Part model, mm, in its own coordinate system. A direction names the side the tool comes from. Coordinates: 2 decimals unless noted, no trailing zeros. Write each loop counter-clockwise with the first axis right and the second up, starting at its lowest first coordinate (ties: lowest second). Pieces come first, ordered by that corner, then holes. Notation, with made-up numbers: (36, -33) - (77, -33) arc R24 ccw to (77, -15) - close; hole circle Ø1 at (44.5, 5). An arc over 180 degrees is marked (long way). Use one line per item in the form item = value. Start each with the question number.
from build123d import *

# Parameters (mm, degrees)
BOSS_EXTRUDE1_START             = -487.984875
SKETCH3_R                       = 24.13
BOSS_EXTRUDE1_DEPTH             = 975.96975
CHAMFER1_SIZE                   = 0.254
BOSS_EXTRUDE3_REACH             = 985.674
SKETCH6_R                       = 24.13
SKETCH6_R_2                     = 22.352
BOSS_EXTRUDE3_DIRECTION_2_REACH = 985.674
BOSS_EXTRUDE2_DEPTH             = 508
BOSS_EXTRUDE2_DEPTH_BACK        = 508
LPATTERN1_COUNT                 = 2
LPATTERN1_PITCH                 = 33.02


with BuildPart() as part:
    # Sketch2 → Revolve1 (revolve)
    with BuildSketch(Plane.XY, mode=Mode.PRIVATE) as revolve1_sk:
        Polygon((-493.7125, 0), (-493.7125, 11.1125), (-495.096875, 11.1125), (-495.096875, 15.712927565), (-489.762875, 15.712927565), (-489.762875, 20.574), (-495.096875, 20.574), (-495.096875, 24.13), (-493.318875, 24.13), (-493.318875, 22.352), (-487.984875, 22.352), (-487.984875, 0), align=None)
    revolve(revolve1_sk.sketch.rotate(Axis((-493.7125, 0, 0), (1, 0, 0)), 180), axis=Axis((-493.7125, 0, 0), (1, 0, 0)))


with BuildPart() as body_2:
    # Mirror2: mirrored copy
    add(part.part.mirror(Plane(origin=(0, 0, 0), x_dir=(0, 0, 1), z_dir=(1, 0, 0))))


with BuildPart() as part_1:
    add(part.part)

    add(body_2.part)  # Boss-Extrude1 merges body 2
    # Sketch3 → Boss-Extrude1 (add)
    with BuildSketch(Plane(origin=(0, 0, 0), x_dir=(0, 0, -1), z_dir=(1, 0, 0)).offset(BOSS_EXTRUDE1_START)):
        with Locations(Location((0, 0, 0), (0, 0, 270))):
            Circle(SKETCH3_R)
    extrude(amount=BOSS_EXTRUDE1_DEPTH)

    # Chamfer1
    chamfer1_edges = [part_1.edges().sort_by_distance(p)[0] for p in [
        (493.318875, 24.13, 0),
        (-493.318875, 24.13, 0),
    ]]
    chamfer(chamfer1_edges, length=CHAMFER1_SIZE)

    # Boss-Extrude3: up to this face of the body (flat: up to its plane)
    boss_extrude3_end = Plane(part_1.part.faces().sort_by_distance((-493.318875, 23.20068474, 0))[0])
    # Sketch6 → Boss-Extrude3 (add, up to the picked face)
    with BuildSketch(Plane.ZY.offset(487.984875), mode=Mode.PRIVATE) as boss_extrude3_sk1:
        with Locations(Location((0, 0, 0), (0, 0, 270))):
            Circle(SKETCH6_R)
        Circle(SKETCH6_R_2, mode=Mode.SUBTRACT)
    boss_extrude3_tool1 = split(extrude(boss_extrude3_sk1.sketch, amount=BOSS_EXTRUDE3_REACH, mode=Mode.PRIVATE), bisect_by=boss_extrude3_end, keep=Keep.BOTH, mode=Mode.PRIVATE)
    add(boss_extrude3_tool1.solids().sort_by(Axis((-487.984875, 23.447501, 0), (-1, 0, 0)))[0])

    # Boss-Extrude3 direction 2: up to this face of the body (flat: up to its plane)
    boss_extrude3_direction_2_end = Plane(part_1.part.faces().sort_by_distance((493.318875, 23.20068474, 0))[0])
    # Sketch6 → Boss-Extrude3 direction 2 (add, up to the picked face)
    with BuildSketch(Plane.ZY.offset(487.984875), mode=Mode.PRIVATE) as boss_extrude3_direction_2_sk1:
        with Locations(Location((0, 0, 0), (0, 0, 270))):
            Circle(SKETCH6_R)
        Circle(SKETCH6_R_2, mode=Mode.SUBTRACT)
    boss_extrude3_direction_2_tool1 = split(extrude(boss_extrude3_direction_2_sk1.sketch, amount=-BOSS_EXTRUDE3_DIRECTION_2_REACH, mode=Mode.PRIVATE), bisect_by=boss_extrude3_direction_2_end, keep=Keep.BOTH, mode=Mode.PRIVATE)
    add(boss_extrude3_direction_2_tool1.solids().sort_by(Axis((-487.984875, 23.447501, 0), (1, 0, 0)))[0])

    # Sketch4 → Boss-Extrude2 (add, two sides: drawn at the far end of the back side and taken through both)
    with BuildSketch(Plane(origin=(0, 0, 0), x_dir=(0, 0, -1), z_dir=(1, 0, 0)).offset(-BOSS_EXTRUDE2_DEPTH_BACK)):
        Polygon((0, 6.415804866), (-5.55625, 3.207902433), (-5.55625, -3.207902433), (0, -6.415804866), (5.55625, -3.207902433), (5.55625, 3.207902433), align=None)
    extrude(amount=BOSS_EXTRUDE2_DEPTH + BOSS_EXTRUDE2_DEPTH_BACK)

    # Sketch5 → Cut-Revolve1 (revolve, cut)
    with BuildSketch(Plane.XY, mode=Mode.PRIVATE) as cut_revolve1_sk:
        with BuildLine():
            Line((-433.38115, 24.8874), (-433.38115, 25.5224))
            Line((-433.38115, 25.5224), (-427.04385, 25.5224))
            Line((-427.04385, 25.5224), (-427.04385, 24.8874))
            ThreePointArc((-427.04385, 24.8874), (-427.60062588, 24.65677588), (-427.83125, 24.1))
            ThreePointArc((-427.83125, 24.1), (-430.2125, 21.71875), (-432.59375, 24.1))
            ThreePointArc((-432.59375, 24.1), (-432.82437412, 24.65677588), (-433.38115, 24.8874))
        make_face()
    cut_revolve1 = revolve(cut_revolve1_sk.sketch.rotate(Axis((-508, 0, 0), (1, 0, 0)), 180), axis=Axis((-508, 0, 0), (1, 0, 0)), mode=Mode.SUBTRACT)

    # LPattern1: Cut-Revolve1 ×2
    with Locations(*[(i * LPATTERN1_PITCH, 0, 0) for i in range(1, LPATTERN1_COUNT)]):
        add(cut_revolve1, mode=Mode.SUBTRACT)


solid = part_1.part
Q1. Mould opens along Y. For faces 1 (the cylindrical face through (-462.532, -23.016, 7.248)), 2 (the flat face through (-495.097, -11, 3)), 3 (the flat face through (-489.763, -14, 8)) say: released by +Y, released by -Y, zero draft, split by the parting line, or undercut.
Q2. Drill centre lines: probe 1 along Z at (x, y) = (494.55, 0); probe 2 along X at (y, z) = (6.5, 7.5); probe 3 along X at (y, z) = (16, -1.5). Where is each one in solid material? Low to high.
Q3. Which spindle directions (+Z, -Z, +X, -X, +Y, -Y) get a long thin tool onto all of the face, cutting with end or side? Do faces 4 (the cylindrical face through (492.47, 2.68, -20.4)), 5 (the cylindrical face through (494.324, -23.016, -7.248)), 6 (the flat face through (-493.712, -5, -3)). Say none if no direction does.
Q4. Pin check, flat tips, straight feed: P1, Ø3, axis at x = 338.5, z = -4.5, coming from the +Y side; P2, Ø15.5, axis at y = 6.5, z = 2.5, coming from the -X side; P3, Ø3, axis at x = -500, y = 1.5, coming from the +Z side; P4, Ø2, axis at x = 134, z = 17, coming from the +Y side. Stop position of each tip, or through.
Q5. Slice it at A-A (x = -288). List the corners of the cut face in (y, z), plus the area to 3 significant figures.
Solution:
q1.face_1 = split by the parting line
q1.face_2 = zero draft
q1.face_3 = undercut
q2.probe_1 = -24.13 to -20.57, -15.71 to -11.11, -5.56 to 5.56, 11.11 to 15.71, 20.57 to 24.13
q2.probe_2 = -493.71 to 493.71
q2.probe_3 = -489.76 to 489.76
q3.face_4 = +X
q3.face_5 = +X, -X
q3.face_6 = -X
q4.P1 = 23.94
q4.P2 = -508
q4.P3 = 5.56
q4.P4 = 18.06
q5.outline = circle Ø48.26 at (0, 0)
q5.area = 1,830 mm2
